Input: part model. Units: mm. Frame: model coordinates. A direction names the side the tool comes from. Give positions to 0.01 mm unless a question says otherwise; leave off trailing zeros. Loops run counter-clockwise (first coordinate to the right, second up) from the corner with the lowest first, then second, coordinate; pieces in that order, holes last. Notation, with made-up numbers: (3.5, -6.75) -> (32.5, -6.75) arc R11 cw to (32.5, -0.75) -> close; hole circle Ø8 at (80.5, -9.75). An arc over 180 degrees is marked (long way). Use CSV: the item, a comma, the result in double quotes.
```python
from build123d import *

# Parameters (mm, degrees)
SKETCH1_R          = 20
EXTRUDE1_DEPTH     = 10
SKETCH2_R          = 2
EXTRUDE2_DEPTH     = 5
SKETCH3_R          = 15
EXTRUDE3_DEPTH     = 110
SKETCH4_W          = 34
SKETCH4_H          = 30
EXTRUDE4_DEPTH     = 2
SKETCH5_W          = 2
SKETCH5_H          = 30
EXTRUDE5_DEPTH     = 120
SKETCH6_W          = 30
SKETCH6_H          = 6
EXTRUDE6_DEPTH     = 30
SKETCH7_R          = 2
CUT_EXTRUDE1_DEPTH = 30


with BuildPart() as part:
    # Sketch1 → Extrude1 (new body)
    with BuildSketch(Plane(origin=(0, 0, 0), x_dir=(1, 0, 0), z_dir=(0, 1, 0))):
        with Locations(Location((0, 0, 0), (0, 0, 270))):
            Circle(SKETCH1_R)
    extrude(amount=EXTRUDE1_DEPTH)

    # Sketch2 → Extrude2 (add)
    with BuildSketch(Plane(origin=(0, 10, 0), x_dir=(1, 0, 0), z_dir=(0, 1, 0))):
        with Locations(Location((0, 0, 0), (0, 0, 270))):
            Circle(SKETCH2_R)
    extrude(amount=EXTRUDE2_DEPTH)

    # Sketch3 → Extrude3 (add)
    with BuildSketch(Plane(origin=(0, 15, 0), x_dir=(1, 0, 0), z_dir=(0, 1, 0))):
        with Locations(Location((0, 0, 0), (0, 0, 270))):
            Circle(SKETCH3_R)
    extrude(amount=EXTRUDE3_DEPTH)

    # Sketch4 → Extrude4 (add)
    with BuildSketch(Plane.XZ.offset(-15)):
        with Locations((2, 0)):
            Rectangle(SKETCH4_W, SKETCH4_H)
    extrude(amount=EXTRUDE4_DEPTH)

    # Sketch5 → Extrude5 (add)
    with BuildSketch(Plane(origin=(0, 15, 0), x_dir=(1, 0, 0), z_dir=(0, 1, 0))):
        with Locations((18, 0)):
            Rectangle(SKETCH5_W, SKETCH5_H)
    extrude(amount=EXTRUDE5_DEPTH)

    # Sketch6 → Extrude6 (add)
    with BuildSketch(Plane.ZY.offset(-17)):
        with Locations((0, 132)):
            Rectangle(SKETCH6_W, SKETCH6_H)
    extrude(amount=EXTRUDE6_DEPTH)

    # Sketch7 → Cut-Extrude1 (cut)
    with BuildSketch(Plane.XY.offset(15)):
        with Locations((0.0001, 132)):
            Circle(SKETCH7_R)
    extrude(amount=-CUT_EXTRUDE1_DEPTH, mode=Mode.SUBTRACT)


solid = part.part
```
1) Section query D-D (y = 35). Return loops of the section in (x, z).
From the geometry:
outline,"circle Ø30 at (0, 0); (17, -15) -> (19, -15) -> (19, 15) -> (17, 15) -> close"
2) Section query B-B (z = 11). Return loops of the section in (x, y), then the cut area to 3 significant figures.
From the geometry:
outline,"(-16.7, 0) -> (16.7, 0) -> (16.7, 10) -> (-16.7, 10) -> close; (-15, 13) -> (19, 13) -> (19, 135) -> (-13, 135) -> (-13, 129) -> (17, 129) -> (17, 15) -> (10.2, 15) -> (10.2, 125) -> (-10.2, 125) -> (-10.2, 15) -> (-15, 15) -> close; hole circle Ø4 at (0, 132)"
area,"3,050 mm^2"
3) Contact query for flat-ended pins moving along their axis: pin 1 (1.6 mm diameter, centred on y = 14.5, z = 7, fed in from -X); pin 2 (3 mm diameter, centred on x = 0, y = 132, fed in from -Z); pin 3 (10 mm diameter, centred on y = 54.5, z = -12, fed in from +X); pin 4 (4 mm diameter, centred on x = -14.5, y = 48, fed in from -Z). Output: stop coordinate, or through.
From the geometry:
pin 1,"stops at x = -15"
pin 2,"passes through"
pin 3,"stops at x = 19"
pin 4,"stops at z = -8.29"
4) Mould query, pull axis X, two halves, no side actions, for faces 4 (the flat face through (17, 71, 0)), 5 (the flat face through (-13, 132, 0)), 6 (the flat face through (17.2, 69.2, 15)). Classes: pulls with the +X half, pulls with the -X half, needs draft (parallel to the pull), parting line crosses it, or undercut.
From the geometry:
face 4,"undercut"
face 5,"pulls with the -X half"
face 6,"needs draft"
5) Ray query, line 1 (Y direction, x = -7, z = 11); line 2 (Y direction, x = 16.5, z = 1); line 3 (X direction, y = 132, z = 3). Return the intervals inside material, ascending.
From the geometry:
line 1,"y = 0 to 10, 13 to 125, 129 to 135"
line 2,"y = 0 to 10, 13 to 15, 129 to 135"
line 3,"x = -13 to -2, 2 to 19"
6) Section query A-A (y = 132). Return loops of the section in (x, z), then the cut area to 3 significant figures.
From the geometry:
outline,"(-13, -15) -> (-2, -15) -> (-2, 15) -> (-13, 15) -> close; (2, -15) -> (19, -15) -> (19, 15) -> (2, 15) -> close"
area,"840 mm^2"
7) Section query C-C (x = 6). Return loops of the section in (y, z).
From the geometry:
outline,"(0, -19.08) -> (10, -19.08) -> (10, 19.08) -> (0, 19.08) -> close; (13, -15) -> (15, -15) -> (15, -13.75) -> (125, -13.75) -> (125, 13.75) -> (15, 13.75) -> (15, 15) -> (13, 15) -> close; (129, -15) -> (135, -15) -> (135, 15) -> (129, 15) -> close"
8) Reachability of faces 1 (the flat face through (0, 125, 0)), 2 (the flat face through (-12, 15, -11)), 3 (the flat face through (-12, 15, 11)) from +Z, -Z, +X, -X, +Y, -Y: full face, straight path, thin tool, end or side. Return the list, or none.
From the geometry:
face 1,"+Z, -Z, -X"
face 2,"-Z, -X"
face 3,"+Z, -X"
